```python
from build123d import *

# Parameters (mm, degrees)
F0_R     = 38.1
F0_R_2   = 19.05
F1_DEPTH = 25.4
F2_W     = 25.4
F2_H     = 8.89
F3_ANGLE = 180
F4_R     = 3.81
F5_SIZE  = 3.81


with BuildPart() as f1:
    # F0 (on Front) → F1 (new body)
    with BuildSketch(Plane.XZ):
        Circle(F0_R)
        Circle(F0_R_2, mode=Mode.SUBTRACT)
    extrude(amount=F1_DEPTH)

    # F2 (on Front) → F3 (revolve)
    with BuildSketch(Plane.XZ):
        with Locations((0.826871, -27.305)):
            Rectangle(F2_W, F2_H)
    revolve(axis=Axis((0.153273, 0, 0), (1, 0, 0)), revolution_arc=F3_ANGLE)

    # F4
    f4_edges = [f1.edges().sort_by_distance(p)[0] for p in [
        (13.526871, 31.75, 0),
        (-11.873129, 31.75, 0),
        (-11.873129, 22.86, 0),
        (13.526871, 22.86, 0),
    ]]
    fillet(f4_edges, radius=F4_R)

    # F5
    f5_edges = [f1.edges().sort_by_distance(p)[0] for p in [
        (-38.1, 0, 0),
        (-38.1, -25.4, 0),
    ]]
    chamfer(f5_edges, length=F5_SIZE)


solid = f1.part
```
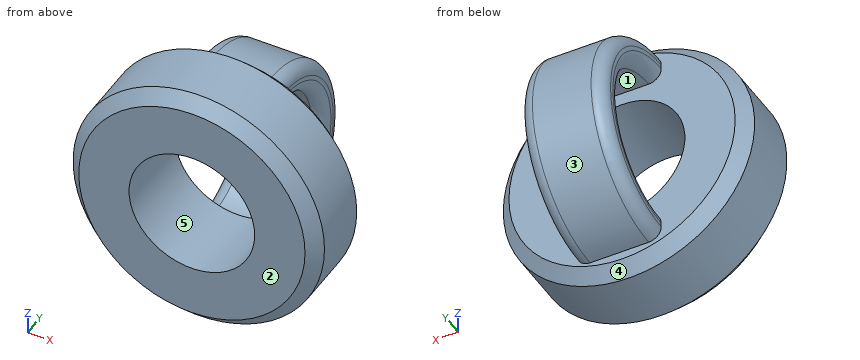
Build history of the part. All positions in model axes, mm. Face numbers are marked on the shaded views. A direction names the side the tool comes from. Give positions to 0.01 mm unless a question says otherwise; leave off trailing zeros. Loops run counter-clockwise (first coordinate to the right, second up) from the corner with the lowest first, then second, coordinate; pieces in that order, holes last. Notation, with made-up numbers: (43.5, 86.25) -> (47.5, 86.25) arc R26 ccw to (47.5, 125.25) -> close; hole circle Ø4 at (-28.75, 20). An arc over 180 degrees is marked (long way). One line per question, with ' | ' between items. Start each with the question number.
1) 3-axis set-ups, long thin cutter, end or side, ignore diameter. For the marked faces 1 and 2: which of +Z, -Z, +X, -X, +Y, -Y reach the whole face in a straight line?
2) Cut at C-C (z = 10.5). Count the separate pieces of the cut face and the enclosed holes in it, plus the area to 3 significant figures.
3) Two-plate mould, pull along X, no slides. Class the marked faces 3, 4 and 5: released by +X, released by -X, zero draft, split by the parting line, or undercut.
4) Pin check, flat tips, straight feed: pin 1 (10 mm diameter, centred on x = 18, y = -4.5, fed in from -Z); pin 2 (22.5 mm diameter, centred on y = 12, z = -12, fed in from +X); pin 3 (14 mm diameter, centred on y = 9, z = 10, fed in from -X); pin 4 (2 mm diameter, centred on x = -1, y = 20.5, fed in from +Z). Stop position of each tip, or through.
5) Cut at A-A (z = 0). Give the cut face in (x, y).
6) Cut at B-B (x = 0). Give the cut face in (y, z), plus the area to 3 significant figures.
7) Probe L1, parallel to Z at x = 0, y = -10; L2, parallel to Y at x = -25.5, z = 19; L3, parallel to X at y = -12, z = 7. List the from-to ranges inside material, lowest first.
Return value:
1) face 1: +X, -X | face 2: +Z, -Z, +X, -X, -Y
2) separate pieces: 3 | enclosed holes: 0 | area: 1,250 mm^2
3) face 3: zero draft | face 4: split by the parting line | face 5: undercut
4) pin 1: z = -35.81 | pin 2: x = 13.53 | pin 3: through | pin 4: z = 25.06
5) outline: (-38.1, -21.59) -> (-34.29, -25.4) -> (-19.05, -25.4) -> (-19.05, 0) -> (-34.29, 0) -> (-38.1, -3.81) -> close; (-11.87, 26.67) arc R3.81 ccw to (-8.06, 22.86) -> (9.72, 22.86) arc R3.81 ccw to (13.53, 26.67) -> (13.53, 27.94) arc R3.81 ccw to (9.72, 31.75) -> (-8.06, 31.75) arc R3.81 ccw to (-11.87, 27.94) -> close; (19.05, -25.4) -> (34.29, -25.4) -> (38.1, -21.59) -> (38.1, -3.81) -> (34.29, 0) -> (19.05, 0) -> close
6) outline: (-25.4, -34.29) -> (-21.59, -38.1) -> (-3.81, -38.1) -> (0, -34.29) -> (0, -31.75) arc R31.75 ccw to (0, 31.75) -> (0, 34.29) -> (-3.81, 38.1) -> (-21.59, 38.1) -> (-25.4, 34.29) -> (-25.4, 19.05) -> (0, 19.05) -> (0, 22.86) arc R22.86 cw to (0, -22.86) -> (0, -19.05) -> (-25.4, -19.05) -> close | area: 1,700 mm^2
7) L1: -38.1 to -19.05, 19.05 to 38.1 | L2: -25.4 to 0 | L3: -37.45 to -17.72, 17.72 to 37.45
